from build123d import *

# Parameters (mm, degrees)
SKETCH1_W           = 40
SKETCH1_H           = 24
BOSS_EXTRUDE1_DEPTH = 1
SKETCH2_W           = 40
SKETCH2_H           = 24
SKETCH2_W_2         = 21
SKETCH2_H_2         = 17.5
SKETCH2_W_3         = 13
SKETCH2_H_3         = 18.5
BOSS_EXTRUDE3_DEPTH = 9
SKETCH3_W           = 1
SKETCH3_H           = 17.5
CUT_EXTRUDE2_DEPTH  = 3
SKETCH4_W           = 10.24
SKETCH4_H           = 11.92
BOSS_EXTRUDE4_DEPTH = 1.21
CUT_EXTRUDE3_DEPTH  = 2
SKETCH8_W           = 4
SKETCH8_H           = 18.5
CUT_EXTRUDE4_DEPTH  = 5
SKETCH11_W          = 24
SKETCH11_H          = 10
CUT_EXTRUDE5_DEPTH  = 2
SKETCH12_W          = 4
SKETCH12_H          = 3
CUT_EXTRUDE6_DEPTH  = 3
BOSS_EXTRUDE5_DEPTH = 3.5
SKETCH14_W          = 1
SKETCH14_H          = 2.25
CUT_EXTRUDE7_DEPTH  = 3
SKETCH15_W          = 38
SKETCH15_H          = 10
CUT_EXTRUDE8_DEPTH  = 0.25
SKETCH16_W          = 38
SKETCH16_H          = 10
CUT_EXTRUDE9_DEPTH  = 0.25
SKETCH17_W          = 18.5
SKETCH17_H          = 4
CUT_EXTRUDE10_DEPTH = 0.25
CUT_EXTRUDE11_DEPTH = 0.25
CUT_EXTRUDE12_DEPTH = 0.25


with BuildPart() as part:
    # Sketch1 → Boss-Extrude1 (new body)
    with BuildSketch(Plane(origin=(0, 0, 0), x_dir=(1, 0, 0), z_dir=(0, 1, 0))):
        with Locations((20, 12)):
            Rectangle(SKETCH1_W, SKETCH1_H)
    extrude(amount=BOSS_EXTRUDE1_DEPTH)

    # Sketch2 → Boss-Extrude3 (add)
    with BuildSketch(Plane(origin=(0, 1, 0), x_dir=(1, 0, 0), z_dir=(0, 1, 0))):
        with Locations((20, 12)):
            Rectangle(SKETCH2_W, SKETCH2_H)
        with Locations((11.5, 12)):
            Rectangle(SKETCH2_W_2, SKETCH2_H_2, mode=Mode.SUBTRACT)
        with Locations((29.5, 12)):
            Rectangle(SKETCH2_W_3, SKETCH2_H_3, mode=Mode.SUBTRACT)
    extrude(amount=BOSS_EXTRUDE3_DEPTH)

    # Sketch3 → Cut-Extrude2 (cut)
    with BuildSketch(Plane(origin=(0, 10, 0), x_dir=(1, 0, 0), z_dir=(0, 1, 0))):
        with Locations((22.5, 12)):
            Rectangle(SKETCH3_W, SKETCH3_H)
    extrude(amount=-CUT_EXTRUDE2_DEPTH, mode=Mode.SUBTRACT)

    # Sketch4 → Boss-Extrude4 (add)
    with BuildSketch(Plane(origin=(0, 1, 0), x_dir=(1, 0, 0), z_dir=(0, 1, 0))):
        with Locations((13.26, 12)):
            Rectangle(SKETCH4_W, SKETCH4_H)
    extrude(amount=BOSS_EXTRUDE4_DEPTH)

    # Sketch5 → Cut-Extrude3 (cut)
    with BuildSketch(Plane(origin=(1, 0, 0), x_dir=(0, 0, -1), z_dir=(1, 0, 0))):
        with BuildLine():
            Line((7.53, 2.25), (7.53, 2.96))
            Line((7.53, 2.96), (7.53, 10))
            Line((7.53, 10), (16.47, 10))
            Line((16.47, 10), (16.47, 2.96))
            Line((16.47, 2.96), (16.47, 2.25))
            ThreePointArc((16.47, 2.25), (16.103883476, 1.366116524), (15.22, 1))
            Line((15.22, 1), (8.78, 1))
            ThreePointArc((8.78, 1), (7.896116524, 1.366116524), (7.53, 2.25))
        make_face()
    extrude(amount=-CUT_EXTRUDE3_DEPTH, mode=Mode.SUBTRACT)

    # Sketch8 → Cut-Extrude4 (cut)
    with BuildSketch(Plane(origin=(0, 10, 0), x_dir=(1, 0, 0), z_dir=(0, 1, 0))):
        with Locations((38, 12)):
            Rectangle(SKETCH8_W, SKETCH8_H)
    extrude(amount=-CUT_EXTRUDE4_DEPTH, mode=Mode.SUBTRACT)

    # Sketch11 → Cut-Extrude5 (cut)
    with BuildSketch(Plane(origin=(40, 0, 0), x_dir=(0, 0, -1), z_dir=(1, 0, 0))):
        with Locations((12, 5)):
            Rectangle(SKETCH11_W, SKETCH11_H)
    extrude(amount=-CUT_EXTRUDE5_DEPTH, mode=Mode.SUBTRACT)

    # Sketch12 → Cut-Extrude6 (cut)
    with BuildSketch(Plane(origin=(0, 10, 0), x_dir=(1, 0, 0), z_dir=(0, 1, 0))):
        with Locations((6, 2.5)):
            Rectangle(SKETCH12_W, SKETCH12_H)
    extrude(amount=-CUT_EXTRUDE6_DEPTH, mode=Mode.SUBTRACT)

    # Sketch13 → Boss-Extrude5 (add)
    with BuildSketch(Plane(origin=(0, 10, 0), x_dir=(1, 0, 0), z_dir=(0, 1, 0))):
        Polygon((1, 16.47), (1, 20.75), (3, 20.75), (3, 15.25), (2, 15.25), (2, 16.25), (0, 16.25), (0, 16.47), align=None)
        Polygon((1, 3.25), (3, 3.25), (3, 8.75), (2, 8.75), (2, 7.75), (0, 7.75), (0, 7.53), (1, 7.53), align=None)
    extrude(amount=-BOSS_EXTRUDE5_DEPTH)

    # Sketch14 → Cut-Extrude7 (cut)
    with BuildSketch(Plane(origin=(0, 10, 0), x_dir=(1, 0, 0), z_dir=(0, 1, 0))):
        with Locations((3.5, 2.125)):
            Rectangle(SKETCH14_W, SKETCH14_H)
    extrude(amount=-CUT_EXTRUDE7_DEPTH, mode=Mode.SUBTRACT)

    # Sketch15 → Cut-Extrude8 (cut)
    with BuildSketch(Plane(origin=(0, 0, -24), x_dir=(-1, 0, 0), z_dir=(0, 0, -1))):
        with Locations((-19, 5)):
            Rectangle(SKETCH15_W, SKETCH15_H)
    extrude(amount=-CUT_EXTRUDE8_DEPTH, mode=Mode.SUBTRACT)

    # Sketch16 → Cut-Extrude9 (cut)
    with BuildSketch(Plane.XY):
        with Locations((19, 5)):
            Rectangle(SKETCH16_W, SKETCH16_H)
    extrude(amount=-CUT_EXTRUDE9_DEPTH, mode=Mode.SUBTRACT)

    # Sketch17 → Cut-Extrude10 (cut)
    with BuildSketch(Plane.ZY.offset(-36)):
        with Locations((-12, 3)):
            Rectangle(SKETCH17_W, SKETCH17_H)
    extrude(amount=-CUT_EXTRUDE10_DEPTH, mode=Mode.SUBTRACT)

    # Sketch18 → Cut-Extrude11 (cut)
    with BuildSketch(Plane(origin=(0, 0, -3.25), x_dir=(-1, 0, 0), z_dir=(0, 0, -1))):
        Polygon((-1, 1), (-1, 6.483981395), (-3, 6.5), (-3, 7), (-8, 7), (-8, 10), (-23, 10), (-23, 7), (-22, 7), (-22, 1), align=None)
    extrude(amount=-CUT_EXTRUDE11_DEPTH, mode=Mode.SUBTRACT)

    # Sketch19 → Cut-Extrude12 (cut)
    with BuildSketch(Plane.XY.offset(-20.75)):
        Polygon((1, 1), (1, 6.5), (3, 6.5), (3, 10), (23, 10), (23, 7), (22, 7), (22, 1), align=None)
    extrude(amount=-CUT_EXTRUDE12_DEPTH, mode=Mode.SUBTRACT)


solid = part.part
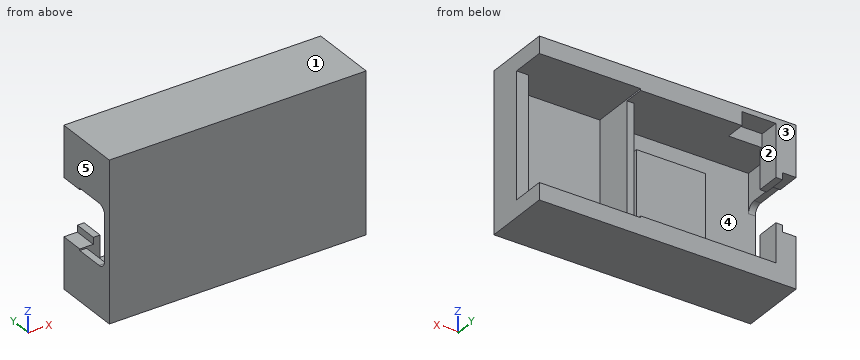
Verification items for the finished model (mm, model axes). Face numbers are marked on the shaded views. A direction names the side the tool comes from. Give positions to 0.01 mm unless a question says otherwise; leave off trailing zeros. Write each loop counter-clockwise with the first axis right and the second up, starting at its lowest first coordinate (ties: lowest second). Pieces come first, ordered by that corner, then holes. Notation, with made-up numbers: M 40,44.25 L 52,44.25 A21 cw 52,61.25 Z; hole C 41.5,64.25 d9. An arc over 180 degrees is marked long. Write item = value, one per line.
(1) Sectioned sample at D-D (x = 22.5). Record the cut outline in (y, z), then the cut area to 3 significant figures.
Found:
outline = M 0,-23.75 L 10,-23.75 L 10,-21 L 7,-21 L 7,-3 L 10,-3 L 10,-0.25 L 0,-0.25 Z
area = 181 mm2
(2) Material ranges on line 1 (Z direction, x = 19.5, y = 7); line 2 (Z direction, x = 28, y = 2.75); line 3 (Y direction, x = 22.5, z = -11.5), recorded low to high.
Found:
line_1 = -23.75 to -21, -3 to -0.25
line_2 = -23.75 to -21.25, -2.75 to -0.25
line_3 = 0 to 7
(3) Draft check along X on the marked faces 3, 4 and 5. Enter one of: released by +X, released by -X, zero draft, split by the parting line, or undercut.
Found:
face_3 = zero draft
face_4 = undercut
face_5 = released by -X
(4) Sectioned sample at C-C (z = -5). Record the cut outline in (x, y).
Found:
outline = M 0,0 L 38,0 L 38,5 L 36.25,5 L 36.25,1 L 23,1 L 23,7 L 22,7 L 22,1 L 1,1 L 1,6.5 L 3,6.5 L 3,10 L 0,10 Z
(5) Access from +Z, -Z, +X, -X, +Y, -Y to the whole of each face (thin tool, end or side, straight path). Record for the marked faces 1 and 2.
Found:
face_1 = +Z, +X, -X, +Y, -Y
face_2 = +Y
(6) Sectioned sample at A-A (y = 7.75). Record the cut outline in (x, z), then the cut area to 3 significant figures.
Found:
outline = M 0,-23.75 L 38,-23.75 L 38,-21.25 L 23,-21.25 L 23,-21 L 3,-21 L 3,-15.25 L 2,-15.25 L 2,-16.25 L 0,-16.25 Z; M 0,-7.75 L 2,-7.75 L 2,-8.75 L 3,-8.75 L 3,-1 L 8,-1 L 8,-3 L 23,-3 L 23,-2.75 L 38,-2.75 L 38,-0.25 L 0,-0.25 Z
area = 222 mm2
(7) Sectioned sample at B-B (y = 2.75). Record the cut outline in (x, z), then the cut area to 3 significant figures.
Found:
outline = M 0,-23.75 L 38,-23.75 L 38,-0.25 L 0,-0.25 L 0,-7.53 L 1,-7.53 L 1,-3 L 22,-3 L 22,-21 L 1,-21 L 1,-16.47 L 0,-16.47 Z; hole M 23,-21.25 L 36.25,-21.25 L 36.25,-2.75 L 23,-2.75 Z
area = 261 mm2
(8) Go/stop test with flat-tipped pins: pin 1 Ø3 at (y, z) = (7, -13.5) entering from -X; pin 2 Ø0.8 at (y, z) = (9, -15.5) entering from -X; pin 3 Ø0.8 at (x, z) = (22.5, -12.5) entering from +Y. Record where each tip stops, or that it passes through.
Found:
pin_1 = 22
pin_2 = 2
pin_3 = 7
